from build123d import *

# Parameters (mm, degrees)
F1_DEPTH = 3.81
F3_R     = 1.27
F4_R     = 0.381
F5_D     = 2.3114
F6_R     = 2.3876
F7_DEPTH = 25.4
F8_R     = 2.3876
F9_DEPTH = 25.4


with BuildPart() as f1:
    # F0 (on Top) → F1 (new body, symmetric)
    with BuildSketch(Plane.XY):
        Polygon((-8.89, 8.89), (-8.89, 0), (-7.62, 0), (-7.62, 7.62), (-1.27, 7.62), (-1.27, 0), (11.43, 0), (11.43, 1.27), (0, 1.27), (0, 8.89), align=None)
    extrude(amount=F1_DEPTH, both=True)

    # F3
    f3_edges = [f1.edges().sort_by_distance(p)[0] for p in [
        (11.43, 0.635, 3.81),
        (11.43, 0.635, -3.81),
        (-8.255, 0, 3.81),
        (-8.255, 0, -3.81),
        (-1.27, 0, 0),
        (0, 8.89, 0),
        (-8.89, 8.89, 0),
    ]]
    fillet(f3_edges, radius=F3_R)

    # F4
    f4_edges = [f1.edges().sort_by_distance(p)[0] for p in [
        (-7.62, 7.62, 0),
        (-1.27, 7.62, 0),
        (0, 1.27, 0),
    ]]
    fillet(f4_edges, radius=F4_R)

    # F5 (through all)
    with Locations(Plane.XZ):
        with Locations((7.62, 0), (3.81, 0)):
            Hole(F5_D / 2)

    # F6 (on face) → F7 (cut)
    with BuildSketch(Plane(origin=(-8.89, 0, 0), x_dir=(0, -1, 0), z_dir=(-1, 0, 0))):
        with Locations((-4.445, 0)):
            Circle(F6_R)
    extrude(amount=-F7_DEPTH, mode=Mode.SUBTRACT)

    # F8 (on face) → F9 (cut)
    with BuildSketch(Plane(origin=(0, 8.89, 0), x_dir=(-1, 0, 0), z_dir=(0, 1, 0))):
        with Locations((4.445, 0)):
            Circle(F8_R)
    extrude(amount=-F9_DEPTH, mode=Mode.SUBTRACT)


solid = f1.part
Here's how the part is built. I have some questions about the finished solid (model axes, mm). A direction names the side the tool comes from. Give positions to 0.01 mm unless a question says otherwise; leave off trailing zeros. Order: outer loops, then holes, each group sorted by start corner. A loop starts at its lowest first (then second) coordinate and runs counter-clockwise, first axis right, second up. Notation, with made-up numbers: (16.25, -35) -> (72.25, -35) arc R17 cw to (72.25, -8) -> close; hole circle Ø11 at (28, -27.5). An arc over 180 degrees is marked (long way). Use a Markdown table: item, result. Add a question column.
Item 1: Imagine slicing it at B-B on z = 1.5. Please give me the cut outline in (x, y), plus the area to 3 significant figures.
Item 2: For faces 1 (the face through (0, 5, 3)), 2 (the face through (-8.246, 0.362, -3.428)), 3 (the face through (-8.246, 0.382, 3.448)), 4 (the face through (-0.888, 0.362, 0.053)), which set-ups out of +Z, -Z, +X, -X, +Y, -Y let a thin tool reach every point of the face, with its end or its side?
Item 3: I need wall thicknesses on line 1 (Z direction, x = 3.81, y = 1); line 2 (Y direction, x = -3.75, z = 2.5); line 3 (Y direction, x = 2, z = -0.5). Which ranges of each line are inside material? Lowest first, please.
Item 4: Will these pins go through, and if not, where does the flat tip stop? pin 1 (3.5 mm diameter, centred on y = 4, z = 1.5, fed in from +X); pin 2 (1 mm diameter, centred on x = 5.5, z = 0, fed in from +Y).
Item 5: Imagine slicing it at D-D on z = 0. Give the number of separate pieces and of enclosed holes in the cut face, plus the area to 3 significant figures.
Item 6: Imagine slicing it at C-C on y = 3.25. Please give me the cut outline in (x, z), plus the area to 3 significant figures.
Item 7: Imagine slicing it at A-A on x = 7.62. Please give me the cut outline in (y, z).
Data:
| question | item | result |
|---|---|---|
| 1 | outline | (-8.89, 0) -> (-7.62, 0) -> (-7.62, 2.59) -> (-8.89, 2.59) -> close; (-8.89, 6.3) -> (-7.62, 6.3) -> (-7.62, 7.24) arc R0.38 cw to (-7.24, 7.62) -> (-6.3, 7.62) -> (-6.3, 8.89) -> (-7.62, 8.89) arc R1.27 ccw to (-8.89, 7.62) -> close; (-2.59, 7.62) -> (-1.65, 7.62) arc R0.38 cw to (-1.27, 7.24) -> (-1.27, 6.3) -> (0, 6.3) -> (0, 7.62) arc R1.27 ccw to (-1.27, 8.89) -> (-2.59, 8.89) -> close; (-1.27, 1.27) arc R1.27 ccw to (0, 0) -> (11.43, 0) -> (11.43, 1.27) -> (0.38, 1.27) arc R0.38 cw to (0, 1.65) -> (0, 2.59) -> (-1.27, 2.59) -> close |
| 1 | area | 30.1 mm² |
| 2 | face 1 | +Z, -Z, +X, +Y |
| 2 | face 2 | -Z, -X, -Y |
| 2 | face 3 | +Z, -X, -Y |
| 2 | face 4 | +Z, -Z, -Y |
| 3 | line 1 | z = -3.81 to -1.16, 1.16 to 3.81 |
| 3 | line 2 | y = 7.62 to 8.89 |
| 3 | line 3 | y = 0 to 1.27 |
| 4 | pin 1 | stops at x = 0 |
| 4 | pin 2 | stops at y = 1.27 |
| 5 | separate pieces | 6 |
| 5 | enclosed holes | 0 |
| 5 | area | 20.2 mm² |
| 6 | outline | (-8.89, -3.81) -> (-7.62, -3.81) -> (-7.62, -2.07) -> (-8.89, -2.07) -> close; (-8.89, 2.07) -> (-7.62, 2.07) -> (-7.62, 3.81) -> (-8.89, 3.81) -> close; (-1.27, -3.81) -> (0, -3.81) -> (0, -2.07) -> (-1.27, -2.07) -> close; (-1.27, 2.07) -> (0, 2.07) -> (0, 3.81) -> (-1.27, 3.81) -> close |
| 6 | area | 8.85 mm² |
| 7 | outline | (0, -3.81) -> (1.27, -3.81) -> (1.27, -1.16) -> (0, -1.16) -> close; (0, 1.16) -> (1.27, 1.16) -> (1.27, 3.81) -> (0, 3.81) -> close |
